Geometry check sheet. Reference: drawing and pictorial views, mm from the part's lowest x, y, z. Round coordinates to 2 decimals unless told otherwise and drop trailing zeros. Write each loop counter-clockwise with the first axis right and the second up, starting at its lowest first coordinate (ties: lowest second). Pieces come first, ordered by that corner, then holes. Notation, with made-up numbers: M 43,77.5 L 77,77.5 A14 cw 77,102.5 Z; hole C -38.5,36.25 d6. An arc over 180 degrees is marked long. Answer in a Markdown table with one row per item. Add a question column.
1. Go/stop test with a flat-tipped pin: pin 1 Ø2 at (x, y) = (5.85, 12.4) entering from -Z. Record where the tip stops, or that it passes through.
2. Sectioned sample at A-A on y = 27.9. Record the cut outline in (x, z), plus the area to 3 significant figures.
3. Material ranges on probe 1 along Y at (x, z) = (5.85, 2.3); probe 2 along Y at (x, z) = (21.35, 1.3); probe 3 along X at (y, z) = (11.5, 0.9), recorded low to high.
4. Sectioned sample at C-C on x = 5.85. Record the cut outline in (y, z).
5. Sectioned sample at D-D on y = 12.4. Record the cut outline in (x, z).
6. Sectioned sample at B-B on x = 21.35. Record the cut outline in (y, z).
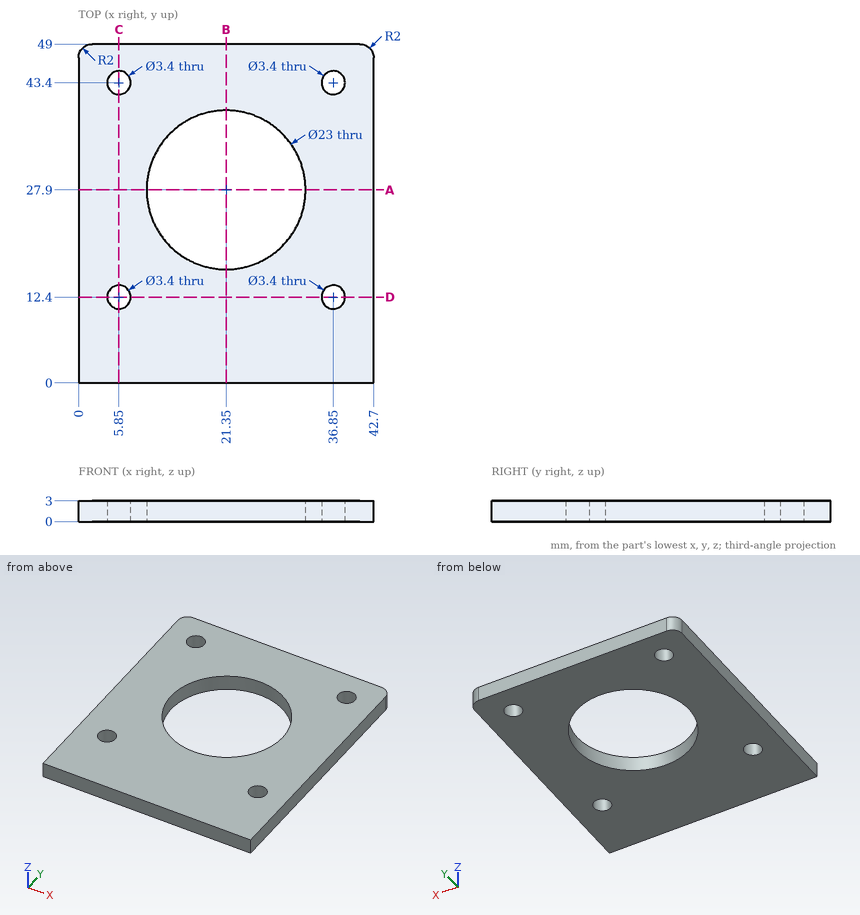
Geometry check:
| question | item | result |
|---|---|---|
| 1 | pin 1 | passes through |
| 2 | outline | M 0,0 L 9.85,0 L 9.85,3 L 0,3 Z; M 32.85,0 L 42.7,0 L 42.7,3 L 32.85,3 Z |
| 2 | area | 59.1 mm2 |
| 3 | probe 1 | y = 0 to 10.7, 14.1 to 41.7, 45.1 to 49 |
| 3 | probe 2 | y = 0 to 16.4, 39.4 to 49 |
| 3 | probe 3 | x = 0 to 4.41, 7.29 to 35.41, 38.29 to 42.7 |
| 4 | outline | M 0,0 L 10.7,0 L 10.7,3 L 0,3 Z; M 14.1,0 L 41.7,0 L 41.7,3 L 14.1,3 Z; M 45.1,0 L 49,0 L 49,3 L 45.1,3 Z |
| 5 | outline | M 0,0 L 4.15,0 L 4.15,3 L 0,3 Z; M 7.55,0 L 35.15,0 L 35.15,3 L 7.55,3 Z; M 38.55,0 L 42.7,0 L 42.7,3 L 38.55,3 Z |
| 6 | outline | M 0,0 L 16.4,0 L 16.4,3 L 0,3 Z; M 39.4,0 L 49,0 L 49,3 L 39.4,3 Z |
